Study the drawing (mm; zero at the part's minimum x, y, z) and answer. A direction names the side the tool comes from. Give positions to 0.01 mm unless a question says otherwise; leave off trailing zeros. Order: outer loops, then holes, each group sorted by start corner. A loop starts at its lowest first (then second) coordinate and runs counter-clockwise, first axis right, second up. Notation, with made-up numbers: (-21.75, 14.5) - (13.25, 14.5) arc R21 cw to (13.25, 41.5) - close; hole circle Ø3 at (27, 37.5). An arc over 180 degrees is marked (long way). Return JSON: item names as keys, results as strings.
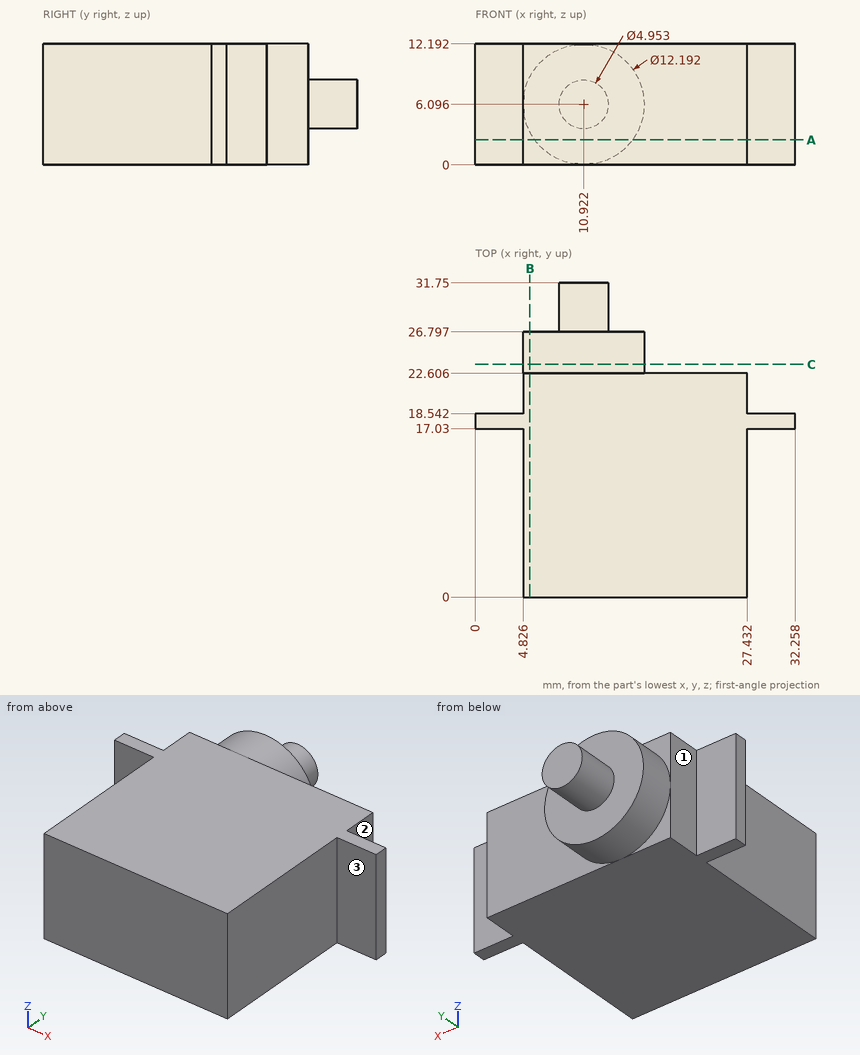
Q1. For the marked faces 1, 2 and 3, determine the directions among +Z, -Z, +X, -X, +Y, -Y from which every point of the face is accessible in a straight line to the end or side of a thin tool.
Values:
{"face 1": "+Z, -Z, -X, +Y", "face 2": "+Z, -Z, +X, +Y", "face 3": "+Z, -Z, +X, -Y"}
Q2. A cutting plane is placed at A-A (z = 2.5). Write down the section's boundary in (x, y), and give its area (3 significant figures).
Values:
{"outline": "(0, 17.03) - (4.83, 17.03) - (4.83, 0) - (27.43, 0) - (27.43, 17.03) - (32.26, 17.03) - (32.26, 18.54) - (27.43, 18.54) - (27.43, 22.61) - (15.84, 22.61) - (15.84, 26.8) - (6, 26.8) - (6, 22.61) - (4.83, 22.61) - (4.83, 18.54) - (0, 18.54) - close", "area": "567 mm²"}
Q3. A cutting plane is placed at C-C (y = 23.5). Write down the section's boundary in (x, z).
Values:
{"outline": "circle Ø12.19 at (10.92, 6.1)"}
Q4. A cutting plane is placed at B-B (x = 5.5). Write down the section's boundary in (y, z).
Values:
{"outline": "(0, 0) - (22.61, 0) - (22.61, 3.31) - (26.8, 3.31) - (26.8, 8.88) - (22.61, 8.88) - (22.61, 12.19) - (0, 12.19) - close"}
Q5. Given pin 1 (4.5 mm diameter, centred on y = 21, z = 3.5, fed in from -X); pin 2 (4 mm diameter, centred on x = 29, z = 4.5, fed in from +Y); pin 3 (6 mm diameter, centred on y = 28, z = 2.5, fed in from -X), each flat-ended and moving along its own axis, determine where each tip first touches the part or whether it passes through.
Values:
{"pin 1": "stops at x = 4.83", "pin 2": "stops at y = 22.61", "pin 3": "stops at x = 4.89"}
Q6. Consider L1, parallel to X at y = 6.5, z = 6; L2, parallel to Y at x = 6, z = 6.25; L3, parallel to Y at x = 17.5, z = 2. Determine where each line is inside the solid, lowest interval first.
Values:
{"L1": "x = 4.83 to 27.43", "L2": "y = 0 to 26.8", "L3": "y = 0 to 22.61"}
